```python
from build123d import *

# Parameters (mm, degrees)
SKETCH_1_W                   = 25.9
SKETCH_1_H                   = 25.9
EXTRUDE_1_DEPTH              = 25.9
HOLE_WIZARD_M3_1_D           = 2.5
SKETCH_7_W                   = 25.9
SKETCH_7_H                   = 9.95
CUT_EXTRUDE_4_DEPTH          = 26.9
FILLET_1_R                   = 2
CUT_EXTRUDE_5_DEPTH          = 1
CUT_EXTRUDE_5_DEPTH_BACK     = 7
FILLET_3_R                   = 1
HOLE_WIZARD_M3_2_D           = 2.5
HOLE_WIZARD_M3_2_ON_FACE_2_D = 2.5


with BuildPart() as part:
    # 草图1 → 凸台-拉伸1 (new body)
    with BuildSketch(Plane.XY):
        Rectangle(SKETCH_1_W, SKETCH_1_H)
    extrude(amount=EXTRUDE_1_DEPTH)

    # M3 螺纹孔1 (through all)
    with Locations(Plane(origin=(12.95, 0, 19.45), x_dir=(0, 0, 1), z_dir=(1, 0, 0))):
        with Locations((0, 0), (-13, 0)):
            Hole(HOLE_WIZARD_M3_1_D / 2)

    # 草图7 → 切除-拉伸4 (cut, through all)
    with BuildSketch(Plane.ZY.offset(12.95)):
        with Locations((12.95, 7.975)):
            Rectangle(SKETCH_7_W, SKETCH_7_H)
        with Locations((12.95, -7.975)):
            Rectangle(SKETCH_7_W, SKETCH_7_H)
    extrude(amount=-CUT_EXTRUDE_4_DEPTH, mode=Mode.SUBTRACT)

    # 圆角1
    fillet_1_edges = [part.edges().sort_by_distance(p)[0] for p in [
        (12.95, 0, 0),
        (-12.95, 0, 0),
        (12.95, 0, 25.9),
        (-12.95, 0, 25.9),
    ]]
    fillet(fillet_1_edges, radius=FILLET_1_R)

    # 草图8 → 切除-拉伸5 (cut, two sides)
    with BuildSketch(Plane(origin=(0, 3, 0), x_dir=(1, 0, 0), z_dir=(0, 1, 0))) as cut_extrude_5_sk:
        Polygon((-6.95, -9.45), (-9.95, -9.45), (-9.95, -16.45), (-6.95, -16.45), (-6.95, -22.4), (6.95, -22.4), (6.95, -16.45), (9.95, -16.45), (9.95, -9.45), (6.95, -9.45), (6.95, -3.5), (-6.95, -3.5), align=None)
    extrude(amount=CUT_EXTRUDE_5_DEPTH, mode=Mode.SUBTRACT)
    extrude(cut_extrude_5_sk.sketch, amount=-CUT_EXTRUDE_5_DEPTH_BACK, mode=Mode.SUBTRACT)

    # 圆角3
    fillet_3_edges = [part.edges().sort_by_distance(p)[0] for p in [
        (6.95, 0, 16.45),
        (-6.95, 0, 22.4),
        (-9.95, 0, 16.45),
        (-9.95, 0, 9.45),
        (-6.95, 0, 3.5),
        (6.95, 0, 9.45),
        (9.95, 0, 9.45),
        (9.95, 0, 16.45),
        (6.95, 0, 22.4),
        (-6.95, 0, 16.45),
        (-6.95, 0, 9.45),
        (6.95, 0, 3.5),
    ]]
    fillet(fillet_3_edges, radius=FILLET_3_R)

    # M3 螺纹孔2 (through all)
    with Locations(Plane(origin=(0, 0, 0), x_dir=(-1, 0, 0), z_dir=(0, 0, -1))):
        with Locations((0, 0)):
            Hole(HOLE_WIZARD_M3_2_D / 2)

    # M3 螺纹孔2 on face 2 (through all)
    with Locations(Plane.XY.offset(25.9)):
        with Locations((0, 0)):
            Hole(HOLE_WIZARD_M3_2_ON_FACE_2_D / 2)


solid = part.part
```
Could you check a few things on this model? Use its own coordinates, in mm. A direction names the side the tool comes from. Give positions to 0.01 mm unless a question says otherwise; leave off trailing zeros. Loops run counter-clockwise (first coordinate to the right, second up) from the corner with the lowest first, then second, coordinate; pieces in that order, holes last. Notation, with made-up numbers: (84.5, 66) - (122.5, 66) arc R17 ccw to (122.5, 81) - close; hole circle Ø5 at (-24, 80.25). An arc over 180 degrees is marked (long way). Answer in a Markdown table with one row per item. Add a question column.
Q1. If we section it at C-C (x = 0): List the corners of the cut face in (y, z) for me.
Q2. If we section it at B-B (z = 21): List the corners of the cut face in (x, y) for me, plus the area to 3 significant figures.
Q3. For pin 1 (3 mm diameter, centred on y = -0.5, z = 20, fed in from -X), with a flat end and sliding along its axis, tell me the tip position at first contact or that it passes through.
Q4. We'd pull the mould along X, two halves only. Please class faces 1 (the face through (-9, 3, 7)), 2 (the face through (1.41, 0.04, 3.5)), 3 (the face through (12.95, 0, 13)): +X half, -X half, draft (parallel to the pull), parting line (faces both ways), or undercut.
Q5. If we section it at A-A (x = -8.25): List the corners of the cut face in (y, z) for me.
Q6. Please list where these lines run through material, in increasing order: L1, parallel to X at y = 0, z = 23.65; L2, parallel to X at y = -0.8, z = 20.75; L3, parallel to Z at x = -11.75, y = -0.55. Write a range as from..to.
Q7. Which directions (+Z, -Z, +X, -X, +Y, -Y) give clear straight access to the entire face, cutting with the end or side of a thin tool? Please do faces 4 (the face through (-9, -3, 7)), 5 (the face through (7.235, -0.042, 9.149)).
The answers:
| question | item | result |
|---|---|---|
| 1 | outline | (-3, 0) - (-1.25, 0) - (-1.25, 3.5) - (-3, 3.5) - close; (-3, 22.4) - (-1.25, 22.4) - (-1.25, 25.9) - (-3, 25.9) - close; (1.25, 0) - (3, 0) - (3, 3.5) - (1.25, 3.5) - close; (1.25, 22.4) - (3, 22.4) - (3, 25.9) - (1.25, 25.9) - close |
| 2 | outline | (-12.95, -3) - (-6.95, -3) - (-6.95, 3) - (-12.95, 3) - close; (6.95, -3) - (12.95, -3) - (12.95, 3) - (6.95, 3) - close |
| 2 | area | 72.0 mm^2 |
| 3 | pin 1 | stops at x = -12.95 |
| 4 | face 1 | draft |
| 4 | face 2 | undercut |
| 4 | face 3 | +X half |
| 5 | outline | (-3, 0) - (3, 0) - (3, 9.45) - (-3, 9.45) - close; (-3, 16.45) - (3, 16.45) - (3, 25.9) - (-3, 25.9) - close; hole circle Ø2.5 at (0, 6.45); hole circle Ø2.5 at (0, 19.45) |
| 6 | L1 | x = -12.95..-1.25, 1.25..12.95 |
| 6 | L2 | x = -12.95..-6.95, 6.95..12.95 |
| 6 | L3 | z = 0.17..5.33, 7.57..18.33, 20.57..25.73 |
| 7 | face 4 | +Z, -Z, +X, -X, -Y |
| 7 | face 5 | +Y, -Y |
